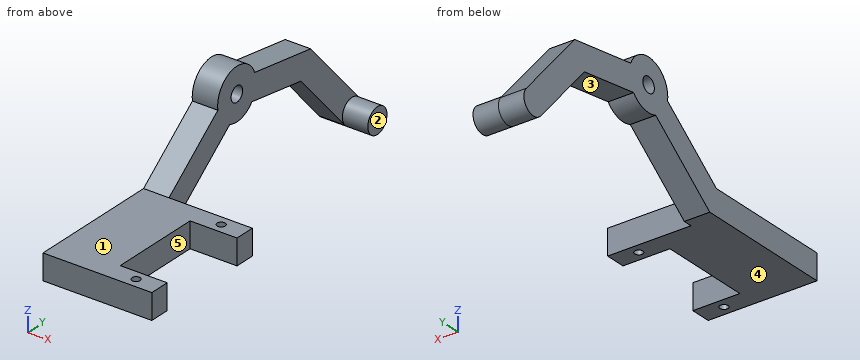
```python
from build123d import *

# Parameters (mm, degrees)
F0_R     = 1.905
F1_DEPTH = 6.35
F2_R     = 3.175
F3_DEPTH = 6.35
F4_W     = 33.274
F4_H     = 6.35
F5_DEPTH = 9.08304
F6_W     = 5.08
F6_H     = 6.35
F7_DEPTH = 11.7348
F8_R     = 1.016
F9_DEPTH = 6.35


with BuildPart() as f1:
    # F0 (on Right) → F1 (new body)
    with BuildSketch(Plane.YZ):
        with BuildLine():
            Line((0, 6.35), (0, 0))
            Line((0, 0), (35.482188, 0))
            Line((35.482188, 0), (53.384841, 14.163968))
            ThreePointArc((53.384841, 14.163968), (57.36122, 13.929732), (60.694788, 16.110049))
            Line((60.694788, 16.110049), (76.933658, 13.673165))
            Line((76.933658, 13.673165), (91.448403, -2.752631))
            ThreePointArc((91.448403, -2.752631), (95.929991, -3.029437), (96.206797, 1.452151))
            Line((96.206797, 1.452151), (80.161637, 19.60986))
            Line((80.161637, 19.60986), (61.637148, 22.389735))
            ThreePointArc((61.637148, 22.389735), (54.09398, 26.202268), (49.444911, 19.143872))
            Line((49.444911, 19.143872), (33.274, 6.35))
            Line((33.274, 6.35), (0, 6.35))
        make_face()
        with Locations((55.7276, 20.066)):
            Circle(F0_R, mode=Mode.SUBTRACT)
    extrude(amount=F1_DEPTH)

    # F2 (on face) → F3 (join)
    with BuildSketch(Plane.YZ.offset(6.35)):
        with Locations((93.8276, -0.65024)):
            Circle(F2_R)
    extrude(amount=F3_DEPTH)

    # F4 (on face) → F5 (join)
    with BuildSketch(Plane.YZ.offset(6.35)):
        with Locations((16.637, 3.175)):
            Rectangle(F4_W, F4_H)
    extrude(amount=F5_DEPTH)

    # F6 (on face) → F7 (join)
    with BuildSketch(Plane.YZ.offset(15.43304)):
        with Locations((2.54, 3.175)):
            Rectangle(F6_W, F6_H)
        with Locations((30.734, 3.175)):
            Rectangle(F6_W, F6_H)
    extrude(amount=F7_DEPTH)

    # F8 (on face) → F9 (cut, through all)
    with BuildSketch(Plane.XY.offset(6.35)):
        with Locations((21.30044, 30.734)):
            Circle(F8_R)
        with Locations((21.30044, 2.54)):
            Circle(F8_R)
    extrude(amount=-F9_DEPTH, mode=Mode.SUBTRACT)


solid = f1.part
```
Part model, mm, in its own coordinate system. Face numbers are marked on the shaded views. A direction names the side the tool comes from. Round coordinates to 2 decimals unless told otherwise and drop trailing zeros. Loops run counter-clockwise (first coordinate to the right, second up) from the corner with the lowest first, then second, coordinate; pieces in that order, holes last.
Item 1: 3-axis set-ups, long thin cutter, end or side, ignore diameter. For the marked faces 1, 2, 3, 4 and 5: which of +Z, -Z, +X, -X, +Y, -Y reach the whole face in a straight line?
Item 2: Cut at D-D, the plane x = 2.75. Give the cut face in (y, z) (3 decimals), then the cut area to 3 significant figures.
Item 3: Cut at A-A, the plane x = 24. Give the cut face in (y, z).
Item 4: Drop flat-ended pins along their axis: P1, Ø14.5, axis at y = 51, z = 14, coming from the +X side; P2, Ø3, axis at y = 11.5, z = 4, coming from the +X side; P3, Ø13.5, axis at x = 16.5, y = 21.5, coming from the +Z side. Give the stop position or say it passes through.
Item 5: Cut at B-B, the plane y = 2.54. Give the cut face in (x, z).
Item 6: Drill centre lines: line 1 (Y direction, x = 22.5, z = 2); line 2 (X direction, y = 2, z = 3); line 3 (Y direction, x = 5.75, z = 3). Where is each one in solid material? Low to high.
Item 7: Cut at C-C, the plane z = 4. Give the cut face in (x, y), then the cut area to 3 significant figures.
A:
1. face 1: +Z, +X, -X, -Y
1. face 2: +Z, -Z, +X, +Y
1. face 3: -Z, +X, -X
1. face 4: -Z, +X, -X, -Y
1. face 5: +Z, -Z, +X
2. outline: (0, 0) - (35.482, 0) - (53.385, 14.164) arc R6.35 ccw to (60.695, 16.11) - (76.934, 13.673) - (91.448, -2.753) arc R3.175 ccw to (96.207, 1.452) - (80.162, 19.61) - (61.637, 22.39) arc R6.35 ccw to (49.445, 19.144) - (33.274, 6.35) - (0, 6.35) - close; hole circle Ø3.81 at (55.728, 20.066)
2. area: 738 mm2
3. outline: (0, 0) - (5.08, 0) - (5.08, 6.35) - (0, 6.35) - close; (28.19, 0) - (33.27, 0) - (33.27, 6.35) - (28.19, 6.35) - close
4. P1: stops at x = 6.35
4. P2: stops at x = 15.43
4. P3: stops at z = 6.35
5. outline: (0, 0) - (20.28, 0) - (20.28, 6.35) - (0, 6.35) - close; (22.32, 0) - (27.17, 0) - (27.17, 6.35) - (22.32, 6.35) - close
6. line 1: y = 0 to 5.08, 28.19 to 33.27
6. line 2: x = 0 to 20.44, 22.16 to 27.17
6. line 3: y = 0 to 39.27, 86.37 to 94.84
7. outline: (0, 0) - (27.17, 0) - (27.17, 5.08) - (15.43, 5.08) - (15.43, 28.19) - (27.17, 28.19) - (27.17, 33.27) - (6.35, 33.27) - (6.35, 40.54) - (0, 40.54) - close; (0, 85.48) - (6.35, 85.48) - (6.35, 93.96) - (0, 93.96) - close; hole circle Ø2.03 at (21.3, 2.54); hole circle Ø2.03 at (21.3, 30.73)
7. area: 726 mm2
